Geometry: final body of the model. Coordinates: model frame, mm. Face numbers are marked on the shaded views. A direction names the side the tool comes from. Give positions to 0.01 mm unless a question says otherwise; leave off trailing zeros. Write each loop counter-clockwise with the first axis right and the second up, starting at its lowest first coordinate (ties: lowest second). Pieces come first, ordered by that corner, then holes.
Q1. Pin query (flat end, axial travel): pin 1 (4 mm diameter, centred on x = 193, z = 73.5, fed in from +Y); pin 2 (3 mm diameter, centred on y = -337.5, z = 57.5, fed in from +X); pin 3 (6 mm diameter, centred on x = 18, z = 57, fed in from +Y); pin 4 (3 mm diameter, centred on x = -408.5, z = 48.5, fed in from -Y). Return the tip coordinate at first contact, or that it passes through.
Q2. Cut plane D-D on y = -161. Return the cut outline in (x, z).
Q3. Reachability of the marked faces 1, 2 and 3 from +Z, -Z, +X, -X, +Y, -Y: full face, straight path, thin tool, end or side. Return the list, or none.
Q4. Line query: L1, parallel to Y at x = -3, z = 41.5; L2, parallel to Z at x = 369.5, y = -749; L3, parallel to X at y = -532, z = 29.5. Output: solid intervals per line, ascending.
Q5. Cut plane C-C on y = -515. Return the cut outline in (x, z).
Q6. Cut plane A-A on x = -87. Return the cut outline in (y, z), plus the area to 3 significant figures.
Q7. Cut plane B-B on z = 60.5. Return the cut outline in (x, y).
```python
from build123d import *

# Parameters (mm, degrees)
F1_DEPTH = 114.3
F2_DEPTH = 25.4
F3_R     = 25.4
F4_R     = 50.8


with BuildPart() as f1:
    # F0 (on Top) → F1 (new body)
    with BuildSketch(Plane.XY):
        with BuildLine():
            Line((127, 0), (-127, 0))
            Line((-127, 0), (-587.281537, -460.281537))
            ThreePointArc((-587.281537, -460.281537), (-603.79962, -543.323551), (-533.4, -590.363073))
            Line((-533.4, -590.363073), (-177.8, -590.363073))
            Line((-177.8, -590.363073), (-177.8, -501.65))
            Line((-177.8, -501.65), (177.8, -501.65))
            Line((177.8, -501.65), (177.8, -590.363073))
            Line((177.8, -590.363073), (533.4, -590.363073))
            ThreePointArc((533.4, -590.363073), (603.79962, -543.323551), (587.281537, -460.281537))
            Line((587.281537, -460.281537), (127, 0))
        make_face()
    extrude(amount=F1_DEPTH)

    # F0 (on Top) → F2 (join)
    with BuildSketch(Plane.XY):
        Polygon((-177.8, -590.363073), (-533.4, -590.363073), (-510.605972, -850.9), (510.605972, -850.9), (533.4, -590.363073), (177.8, -590.363073), (177.8, -501.65), (-177.8, -501.65), align=None)
    extrude(amount=F2_DEPTH)

    # F3
    f3_edges = [f1.edges().sort_by_distance(p)[0] for p in [
        (-177.8, -590.363073, 69.85),
        (177.8, -590.363073, 69.85),
        (177.8, -501.65, 69.85),
        (-177.8, -501.65, 69.85),
    ]]
    fillet(f3_edges, radius=F3_R)

    # F4
    f4_edges = [f1.edges().sort_by_distance(p)[0] for p in [
        (-127, 0, 57.15),
        (127, 0, 57.15),
        (-510.605972, -850.9, 12.7),
        (510.605972, -850.9, 12.7),
    ]]
    fillet(f4_edges, radius=F4_R)


solid = f1.part
```
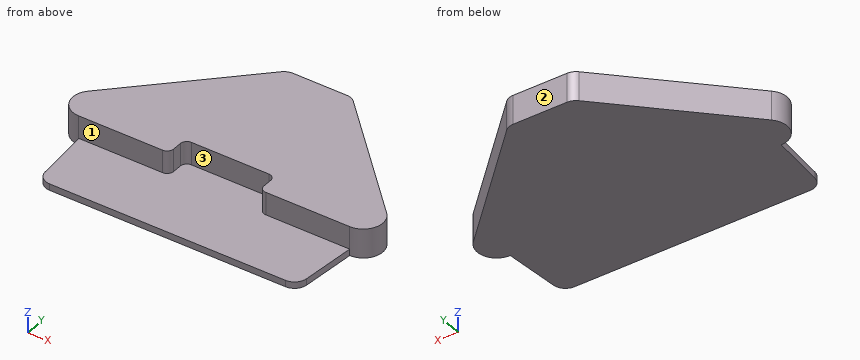
Data:
1. pin 1: stops at y = -64
1. pin 2: stops at x = 466
1. pin 3: stops at y = 0
1. pin 4: stops at y = -590.36
2. outline: (-288, 0) - (288, 0) - (288, 114.3) - (-288, 114.3) - close
3. face 1: +Z, +X, -X, -Y
3. face 2: +Z, -Z, +X, -X, +Y
3. face 3: +Z, -Y
4. L1: y = -501.65 to 0
4. L2: z = 0 to 25.4
4. L3: x = -607.48 to -177.8, 177.8 to 607.48
5. outline: (-609.6, 0) - (609.6, 0) - (609.6, 114.3) - (174.76, 114.3) - (174.76, 25.4) - (-174.76, 25.4) - (-174.76, 114.3) - (-609.6, 114.3) - close
6. outline: (-850.9, 0) - (0, 0) - (0, 114.3) - (-501.65, 114.3) - (-501.65, 25.4) - (-850.9, 25.4) - close
6. area: 66,200 mm2
7. outline: (-587.28, -460.28) arc R76.2 ccw to (-533.4, -590.36) - (-203.2, -590.36) arc R25.4 ccw to (-177.8, -564.96) - (-177.8, -527.05) arc R25.4 cw to (-152.4, -501.65) - (152.4, -501.65) arc R25.4 cw to (177.8, -527.05) - (177.8, -564.96) arc R25.4 ccw to (203.2, -590.36) - (533.4, -590.36) arc R76.2 ccw to (587.28, -460.28) - (141.88, -14.88) arc R50.8 ccw to (105.96, 0) - (-105.96, 0) arc R50.8 ccw to (-141.88, -14.88) - close
